For this review, take the finished solid that the model builds, in its own axes (mm). Face numbers are marked on the shaded views. A direction names the side the tool comes from. Round coordinates to 2 decimals unless told otherwise and drop trailing zeros. Write each loop counter-clockwise with the first axis right and the second up, starting at its lowest first coordinate (ties: lowest second). Pieces come first, ordered by that corner, then holes. Notation, with made-up numbers: M 33.25,11.5 L 42.25,11.5 A13 ccw 42.25,19.5 Z; hole C 31.25,-33 d1. An arc over 180 degrees is marked long. Use one line per item in the form item = value. Start each with the question number.
Item 1: Add section D-D (y = 2). State the section outline as (x, z) points, and give its area (3 significant figures).
Item 2: For line 1 (Z direction, x = 0, y = -0.5); line 2 (Z direction, x = 0, y = 6.25); line 3 (Z direction, x = 3.5, y = -2), list the stretches that pass through material, from the lowest coordinate up. Write a range as [from, to].
Item 3: Add section A-A (x = 0). State the section outline as (y, z) points.
Item 4: Add section B-B (z = 11.75). State the section outline as (x, y) points.
Item 5: Add section C-C (z = 5.25). State the section outline as (x, y) points, and give its area (3 significant figures).
Item 6: For P1, Ø2.5, axis at y = 0.5, z = 4.5, coming from the +X side; P2, Ø1.8, axis at x = 6, z = 8.5, coming from the -Y side; P3, Ø1.5, axis at x = -2, z = 1, coming from the +Y side, all flat-tipped, find the tip position at first contact; note any pin that passes through.
Item 7: For the marked faces 3, 4 and 5, list the 3-axis set-ups (+Z, -Z, +X, -X, +Y, -Y) from which the entire face can be reached by the end or side of a thin tool; tool diameter is ignored.
Item 8: Draft analysis for pull direction Y (two halves, no side actions). For the marked faces 1 and 2, state which applies: released by +Y, released by -Y, zero draft, split by the parting line, or undercut.
from build123d import *
from build123d import SkipClean  # not in build123d's __all__

# Parameters (mm, degrees)
F0_R           = 8
F1_DEPTH       = 3
F2_R           = 8
F3_DEPTH       = 9
F4_R           = 3
F5_DEPTH       = 12.5
F7_DEPTH       = 10
F8_W           = 4.7
F8_H           = 4.7
F9_DEPTH       = 3
F10_R          = 2.5
F11_DEPTH      = 8.001
F11_DEPTH_BACK = 25


# Not quite as in the source:
# - after a boolean that leaves OpenCascade's solid faulty, fix() repairs it


with BuildPart() as f1:
    # F0 (on Top) → F1 (new body)
    with BuildSketch(Plane.XY):
        Circle(F0_R)
    extrude(amount=F1_DEPTH)

    # F2 (on face) → F3 (join)
    with BuildSketch(Plane(origin=(0, 0, 0), x_dir=(1, 0, 0), z_dir=(0, 0, -1))):
        Circle(F2_R)
    extrude(amount=F3_DEPTH)

    # F4 (on face) → F5 (cut, symmetric)
    with BuildSketch(Plane.XY.offset(3)):
        with Locations((-8, 0)):
            Circle(F4_R)
        with Locations((8, 0)):
            Circle(F4_R)
    extrude(amount=F5_DEPTH, both=True, mode=Mode.SUBTRACT)

    # F6 (on face) → F7 (join)
    with BuildSketch(Plane.XY.offset(3)):
        with BuildLine():
            ThreePointArc((-7.4375, -2.9467938085), (0, -8), (7.4375, -2.9467938085))
            Line((7.4375, -2.9467938085), (3.75, -2.9467938085))
            Line((3.75, -2.9467938085), (3.75, -3.25))
            Line((3.75, -3.25), (-3.75, -3.25))
            Line((-3.75, -3.25), (-3.75, -2.9467938085))
            Line((-3.75, -2.9467938085), (-7.4375, -2.9467938085))
        make_face()
        with BuildLine():
            Line((-3.75, 3.25), (3.75, 3.25))
            Line((3.75, 3.25), (3.75, 2.9467938085))
            Line((3.75, 2.9467938085), (7.4375, 2.9467938085))
            ThreePointArc((7.4375, 2.9467938085), (0, 8), (-7.4375, 2.9467938085))
            Line((-7.4375, 2.9467938085), (-3.75, 2.9467938085))
            Line((-3.75, 2.9467938085), (-3.75, 3.25))
        make_face()
    extrude(amount=F7_DEPTH)

    # F8 (on face) → F9 (join)
    with BuildSketch(Plane.XY.offset(3)):
        with BuildLine():
            ThreePointArc((-7.4375, 2.9467938085), (-5, 0), (-7.4375, -2.9467938085))
            Line((-7.4375, -2.9467938085), (-3.75, -2.9467938085))
            Line((-3.75, -2.9467938085), (-3.75, -3.25))
            Line((-3.75, -3.25), (3.75, -3.25))
            Line((3.75, -3.25), (3.75, -2.9467938085))
            Line((3.75, -2.9467938085), (7.4375, -2.9467938085))
            ThreePointArc((7.4375, -2.9467938085), (5, 0), (7.4375, 2.9467938085))
            Line((7.4375, 2.9467938085), (3.75, 2.9467938085))
            Line((3.75, 2.9467938085), (3.75, 3.25))
            Line((3.75, 3.25), (-3.75, 3.25))
            Line((-3.75, 3.25), (-3.75, 2.9467938085))
            Line((-3.75, 2.9467938085), (-7.4375, 2.9467938085))
        make_face()
        Rectangle(F8_W, F8_H, mode=Mode.SUBTRACT)
    with SkipClean():  # cleaning this boolean's faces spoils the solid; the shape is the same uncleaned
        extrude(amount=F9_DEPTH)

    # F10 (on Front) → F11 (cut, two sides)
    with BuildSketch(Plane.XZ) as f11_sk:
        with Locations((0, -4.5)):
            Circle(F10_R)
    extrude(amount=-F11_DEPTH, mode=Mode.SUBTRACT)
    extrude(f11_sk.sketch, amount=F11_DEPTH_BACK, mode=Mode.SUBTRACT)

    add(f1.part.fix(), mode=Mode.REPLACE)


solid = f1.part
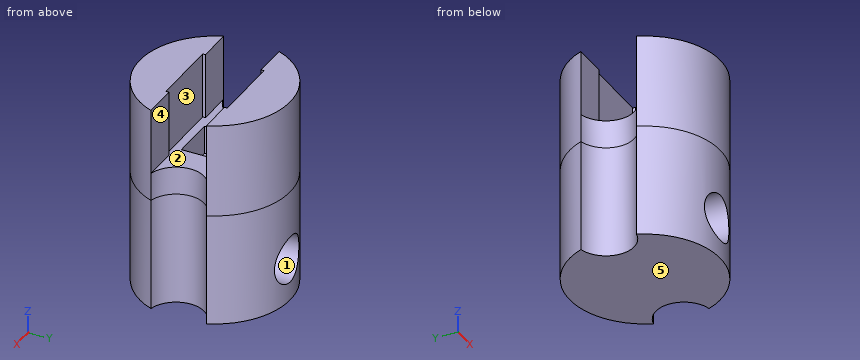
Calculated:
q1.outline = M -5.76,-9 L 5.76,-9 L 5.76,6 L 2.35,6 L 2.35,3 L -2.35,3 L -2.35,6 L -5.76,6 Z; hole C 0,-4.5 d5
q1.area = 139 mm^2
q2.line_1 = [-9, -7], [-2, 3]
q2.line_2 = [-9, -7], [-2, 13]
q2.line_3 = [-9, 6]
q3.outline = M -8,-9 L 8,-9 L 8,-7 L -8,-7 Z; M -8,-2 L 8,-2 L 8,13 L 3.25,13 L 3.25,6 L 2.35,6 L 2.35,3 L -2.35,3 L -2.35,6 L -3.25,6 L -3.25,13 L -8,13 Z
q4.outline = M -7.44,-2.95 A8 ccw 7.44,-2.95 L 3.75,-2.95 L 3.75,-3.25 L -3.75,-3.25 L -3.75,-2.95 Z; M -7.44,2.95 L -3.75,2.95 L -3.75,3.25 L 3.75,3.25 L 3.75,2.95 L 7.44,2.95 A8 ccw Z
q5.outline = M -7.44,-2.95 A8 ccw 7.44,-2.95 A3 cw 7.44,2.95 A8 ccw -7.44,2.95 A3 cw Z; hole M -2.35,-2.35 L 2.35,-2.35 L 2.35,2.35 L -2.35,2.35 Z
q5.area = 153 mm^2
q6.P1 = 5.56
q6.P2 = -6.16
q6.P3 = 7.9
q7.face_3 = +Z
q7.face_4 = +Z, +X, -X
q7.face_5 = -Z, +X, -X, +Y, -Y
q8.face_1 = zero draft
q8.face_2 = undercut
